Check sheet for the drawn part. Datum: minimum x, y, z corner. Units: mm. A direction names the side the tool comes from. Round coordinates to 2 decimals unless told otherwise and drop trailing zeros. Loops run counter-clockwise (first coordinate to the right, second up) from the corner with the lowest first, then second, coordinate; pieces in that order, holes last.
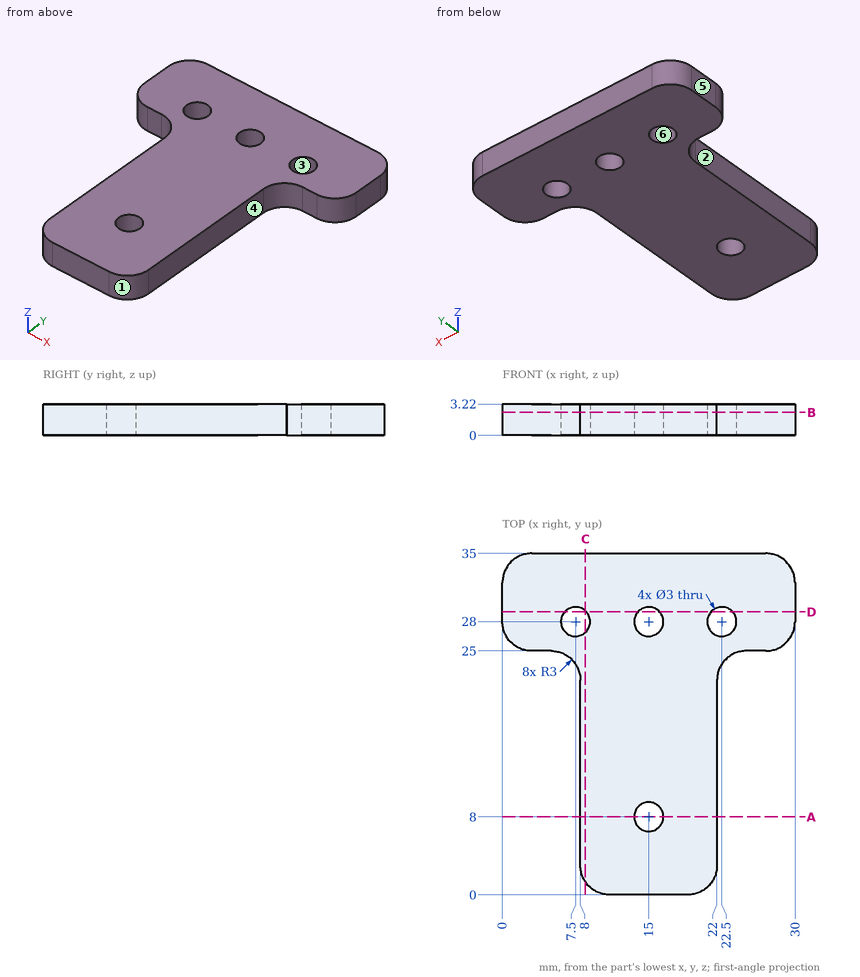
1) Sectioned sample at A-A, the plane y = 8. Record the cut outline in (x, z).
Report:
outline: (8, 0) - (13.5, 0) - (13.5, 3.22) - (8, 3.22) - close; (16.5, 0) - (22, 0) - (22, 3.22) - (16.5, 3.22) - close
2) Scan lines: line 1 along Y through (x, z) = (15, 1.1); line 2 along X through (y, z) = (3.5, 1.05); line 3 along Y through (x, z) = (22.25, 1.8). Record each from-to range of solid material in increasing order.
Report:
line 1: y = 0 to 6.5, 9.5 to 26.5, 29.5 to 35
line 2: x = 8 to 22
line 3: y = 23.2 to 26.52, 29.48 to 35
3) Sectioned sample at B-B, the plane z = 2.35. Record the cut outline in (x, y).
Report:
outline: (0, 28) arc R3 ccw to (3, 25) - (5, 25) arc R3 cw to (8, 22) - (8, 3) arc R3 ccw to (11, 0) - (19, 0) arc R3 ccw to (22, 3) - (22, 22) arc R3 cw to (25, 25) - (27, 25) arc R3 ccw to (30, 28) - (30, 32) arc R3 ccw to (27, 35) - (3, 35) arc R3 ccw to (0, 32) - close; hole circle Ø3 at (7.5, 28); hole circle Ø3 at (15, 8); hole circle Ø3 at (15, 28); hole circle Ø3 at (22.5, 28)
4) Sectioned sample at D-D, the plane y = 29. Record the cut outline in (x, z), then the cut area to 3 significant figures.
Report:
outline: (0, 0) - (6.38, 0) - (6.38, 3.22) - (0, 3.22) - close; (8.62, 0) - (13.88, 0) - (13.88, 3.22) - (8.62, 3.22) - close; (16.12, 0) - (21.38, 0) - (21.38, 3.22) - (16.12, 3.22) - close; (23.62, 0) - (30, 0) - (30, 3.22) - (23.62, 3.22) - close
area: 75.0 mm2
5) Access from +Z, -Z, +X, -X, +Y, -Y to the whole of each face (thin tool, end or side, straight path). Record for the marked faces 1 and 2.
Report:
face 1: +Z, -Z, +X, -Y
face 2: +Z, -Z, -X, -Y
6) Mould release check, pull along X, two halves, no side actions. Record for the marked faces 3, 4, 5 and 6: +X half, -X half, draft (parallel to the pull), parting line (faces both ways), or undercut.
Report:
face 3: undercut
face 4: +X half
face 5: -X half
face 6: undercut
7) Sectioned sample at C-C, the plane x = 8.5. Record the cut outline in (y, z), then the cut area to 3 significant figures.
Report:
outline: (1.34, 0) - (26.88, 0) - (26.88, 3.22) - (1.34, 3.22) - close; (29.12, 0) - (35, 0) - (35, 3.22) - (29.12, 3.22) - close
area: 101 mm2
8) Gauge pin test, flat end, axial feed: pin 1 (1 mm diameter, centred on x = 4, z = 1.5, fed in from -Y). Record the tip position at first contact, or that the pin passes through.
Report:
pin 1: stops at y = 25
